The listing builds one solid part. Answer for the finished solid, in the listing's coordinates (mm). Coordinates: 2 decimals unless noted, no trailing zeros. Loops run counter-clockwise (first coordinate to the right, second up) from the corner with the lowest first, then second, coordinate; pieces in that order, holes last. Notation, with made-up numbers: (54, 29) - (112, 29) arc R8 cw to (112, 44) - close; hole circle Ø11 at (81, -9.5). An arc over 180 degrees is marked (long way). Write each question's results on one line, items separated by ' | '. Start each with the question number.
(1) Find section A-A on x = -12.5. Determine the outline of the cut face in (y, z), then the cut area to 3 significant figures.
(2) Find section B-B on z = 1.45. Determine the outline of the cut face in (x, y), then the cut area to 3 significant figures.
(3) Consider line 1 (Y direction, x = -25, z = 0.85); line 2 (Y direction, x = 2.5, z = 2.1). Determine where each line is inside the solid, lowest interval first. Write a range as from..to.
from build123d import *

# Parameters (mm, degrees)
F0_W       = 152.4
F0_H       = 83.058
F0_W_2     = 76.708
F0_H_2     = 3.048
F1_DEPTH   = 2.54
F2_SIZE2   = 2.0935777936
F2_SIZE    = 0.762
F3_SIZE2   = 2.0935777936
F3_SIZE    = 0.762
F3_2_SIZE2 = 2.0935777936
F3_2_SIZE  = 0.762


with BuildPart() as f1:
    # F0 (on Top) → F1 (new body)
    with BuildSketch(Plane.XY):
        with Locations((0, -6.985)):
            Rectangle(F0_W, F0_H)
        Rectangle(F0_W_2, F0_H_2, mode=Mode.SUBTRACT)
    extrude(amount=F1_DEPTH)

    # F2
    f2_edges = [f1.edges().sort_by_distance(p)[0] for p in [
        (0, 1.524, 0),
    ]]
    f2_side = f1.faces().sort_by_distance((0, -7.116448, 0))[0]
    chamfer(f2_edges, length=F2_SIZE, length2=F2_SIZE2, reference=f2_side)

    # F3
    f3_edges = [f1.edges().sort_by_distance(p)[0] for p in [
        (0, -1.524, 2.54),
    ]]
    f3_side = f1.faces().sort_by_distance((0, -7.116448, 2.54))[0]
    chamfer(f3_edges, length=F3_SIZE, length2=F3_SIZE2, reference=f3_side)

    # F3#2
    f3_2_edges = [f1.edges().sort_by_distance(p)[0] for p in [
        (-76.2, -6.985, 0),
    ]]
    f3_2_side = f1.faces().sort_by_distance((-76.2, -6.985, 1.27))[0]
    chamfer(f3_2_edges, length=F3_2_SIZE, length2=F3_2_SIZE2, reference=f3_2_side)


solid = f1.part
Values:
1) outline: (-48.51, 0) - (-1.52, 0) - (-1.52, 0.45) - (-2.29, 2.54) - (-48.51, 2.54) - close; (1.52, 2.09) - (2.29, 0) - (34.54, 0) - (34.54, 2.54) - (1.52, 2.54) - close | area: 202 mm²
2) outline: (-76.2, -48.51) - (76.2, -48.51) - (76.2, 34.54) - (-76.2, 34.54) - close; hole (-38.35, -1.89) - (38.35, -1.89) - (38.35, 1.76) - (-38.35, 1.76) - close | area: 12,400 mm²
3) line 1: y = -48.51..-1.67, 1.98..34.54 | line 2: y = -48.51..-2.13, 1.52..34.54
